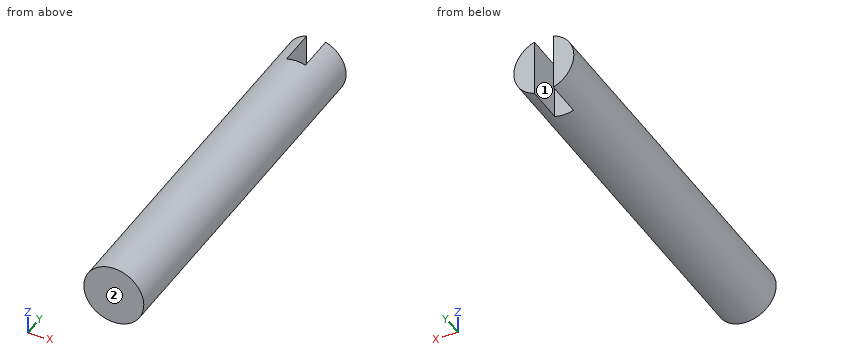
```python
from build123d import *

# Parameters (mm, degrees)
SKETCH1_R           = 1.587
BOSS_EXTRUDE1_DEPTH = 20
CUT_EXTRUDE1_START  = -2
CUT_EXTRUDE1_DEPTH  = 2


with BuildPart() as part:
    # Sketch1 → Boss-Extrude1 (new body)
    with BuildSketch(Plane(origin=(0, 0, 0), x_dir=(1, 0, 0), z_dir=(0, 1, 0))):
        with Locations(Location((0, 0, 0), (0, 0, 270))):
            Circle(SKETCH1_R)
    extrude(amount=BOSS_EXTRUDE1_DEPTH)

    # Sketch2 → Cut-Extrude1 (cut)
    with BuildSketch(Plane(origin=(0, 20, 0), x_dir=(1, 0, 0), z_dir=(0, 1, 0)).offset(CUT_EXTRUDE1_START)):
        with BuildLine():
            ThreePointArc((0.5, 1.506176948), (0.253245121, 1.566663942), (0, 1.587))
            ThreePointArc((0, 1.587), (-0.253245121, 1.566663942), (-0.5, 1.506176948))
            Line((-0.5, 1.506176948), (-0.5, -1.506176948))
            ThreePointArc((-0.5, -1.506176948), (-0.253245121, -1.566663942), (0, -1.587))
            ThreePointArc((0, -1.587), (0.253245121, -1.566663942), (0.5, -1.506176948))
            Line((0.5, -1.506176948), (0.5, 1.506176948))
        make_face()
    extrude(amount=CUT_EXTRUDE1_DEPTH, mode=Mode.SUBTRACT)


solid = part.part
```
Input: part model. Units: mm. Frame: model coordinates. Face numbers are marked on the shaded views. A direction names the side the tool comes from. Give positions to 0.01 mm unless a question says otherwise; leave off trailing zeros. Loops run counter-clockwise (first coordinate to the right, second up) from the corner with the lowest first, then second, coordinate; pieces in that order, holes last. Notation, with made-up numbers: M 37,48 L 75,48 A15 ccw 75,55 Z; hole C 25.5,-1 d2. An arc over 180 degrees is marked long. Answer as CSV lines item,"result". Start each with the question number.
1. Section D-D on z = 1. Return loops of the section in (x, y), plus the area to 3 significant figures.
2. Section A-A on z = 0. Return loops of the section in (x, y).
3. Section B-B on x = 0. Return loops of the section in (y, z), plus the area to 3 significant figures.
4. Section C-C on y = 4.25. Return loops of the section in (x, z), plus the area to 3 significant figures.
5. Pin query (flat end, axial travel): P1, Ø1.5, axis at y = 17.5, z = 1, coming from the -X side; P2, Ø0.6, axis at y = 18.5, z = 0.5, coming from the +X side. Return the tip coordinate at first contact, or that it passes through.
6. Reachability of the marked faces 1 and 2 from +Z, -Z, +X, -X, +Y, -Y: full face, straight path, thin tool, end or side. Return the list, or none.
7. Line query: L1, parallel to X at y = 12.25, z = 0.1; L2, parallel to Y at x = -0.25, z = -1.2; L3, parallel to Z at x = 0.5, y = 2. Output: solid intervals per line, ascending.
Computed values:
1,outline,"M -1.23,0 L 1.23,0 L 1.23,20 L 0.5,20 L 0.5,18 L -0.5,18 L -0.5,20 L -1.23,20 Z"
1,area,"47.3 mm²"
2,outline,"M -1.59,0 L 1.59,0 L 1.59,20 L 0.5,20 L 0.5,18 L -0.5,18 L -0.5,20 L -1.59,20 Z"
3,outline,"M 0,-1.59 L 18,-1.59 L 18,1.59 L 0,1.59 Z"
3,area,"57.1 mm²"
4,outline,"C 0,0 d3.17"
4,area,"7.91 mm²"
5,P1,"stops at x = -1.57"
5,P2,"stops at x = 1.57"
6,face 1,"+Z, -Z, +Y"
6,face 2,"+Z, -Z, +X, -X, -Y"
7,L1,"x = -1.58 to 1.58"
7,L2,"y = 0 to 18"
7,L3,"z = -1.51 to 1.51"
